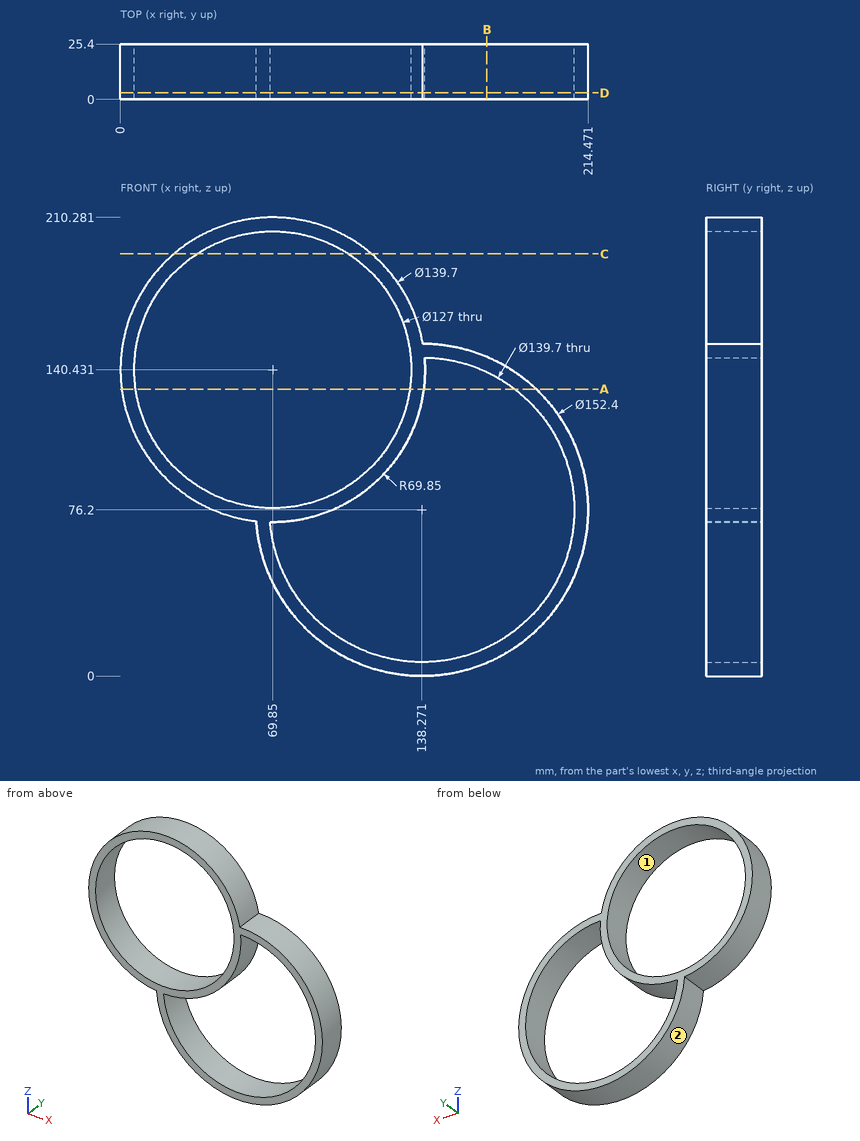
The figure shows three views and two pictorial views of one solid part (mm, origin at its lowest corner). Answer the questions. Give positions to 0.01 mm unless a question says otherwise; leave off trailing zeros. Loops run counter-clockwise (first coordinate to the right, second up) from the corner with the lowest first, then second, coordinate; pieces in that order, holes last. Notation, with made-up numbers: (85, 56) - (133, 56) arc R15 cw to (133, 74) - close; hole circle Ø10 at (33, 67.5). An arc over 180 degrees is marked (long way). Answer in a Markdown table with one row per item.
(1) Section A-A (z = 131.5) is taken. Give the vertices of the cut face in (x, y) (1 decimal).
Results list:
| item | result |
|---|---|
| outline | (0.6, 0) - (7, 0) - (7, 25.4) - (0.6, 25.4) - close; (132.7, 0) - (139.1, 0) - (139.1, 25.4) - (132.7, 25.4) - close; (180.9, 0) - (190.7, 0) - (190.7, 25.4) - (180.9, 25.4) - close |
(2) Consider L1, parallel to Z at x = 126, y = 7 (1 decimal); L2, parallel to X at y = 1.5, z = 119 (1 decimal); L3, parallel to Z at x = 78.5, y = 6.5 (1 decimal). Determine where each line is inside the solid, lowest interval first. Write a range as [from, to].
Results list:
| item | result |
|---|---|
| L1 | z = [1, 7.4], [98.9, 110.8], [170.1, 182] |
| L2 | x = [3.4, 10.1], [129.6, 136.3], [193.5, 201.3] |
| L3 | z = [28.9, 40.1], [71.1, 77.5], [203.3, 209.7] |
(3) Section C-C (z = 193.5) is taken. Give the vertices of the cut face in (x, y).
Results list:
| item | result |
|---|---|
| outline | (24.43, 0) - (34.98, 0) - (34.98, 25.4) - (24.43, 25.4) - close; (104.72, 0) - (115.27, 0) - (115.27, 25.4) - (104.72, 25.4) - close |
(4) Flat-ended cylindrical pins translate along their axes: pin 1 Ø3 at (x, y) = (98.5, 16.5) entering from +Z; pin 2 Ø10 at (y, z) = (19.5, 79) entering from +X; pin 3 Ø6 at (x, y) = (149.5, 18.5) entering from -Z (1 decimal). Find the tip coordinate at first contact, or state that the pin passes through.
Results list:
| item | result |
|---|---|
| pin 1 | stops at z = 204.79 |
| pin 2 | stops at x = 214.47 |
| pin 3 | stops at z = 0.4 |
(5) Section B-B (x = 168) is taken. Give the vertices of the cut face in (y, z).
Results list:
| item | result |
|---|---|
| outline | (0, 6.04) - (25.4, 6.04) - (25.4, 12.99) - (0, 12.99) - close; (0, 139.41) - (25.4, 139.41) - (25.4, 146.36) - (0, 146.36) - close |
(6) Section D-D (y = 3) is taken. State how many separate pieces and enclosed holes the cut face has.
Results list:
| item | result |
|---|---|
| separate pieces | 1 |
| enclosed holes | 2 |
(7) For a pull along Z with two mould halves and no side action, classify the marked faces 1 and 2 as pulls with the +Z half, pulls with the -Z half, needs draft (parallel to the pull), parting line crosses it, or undercut.
Results list:
| item | result |
|---|---|
| face 1 | undercut |
| face 2 | parting line crosses it |
